CAD build for the part. Positions are in the model's coordinates, mm. A direction names the side the tool comes from. Give positions to 0.01 mm unless a question says otherwise; leave off trailing zeros. Loops run counter-clockwise (first coordinate to the right, second up) from the corner with the lowest first, then second, coordinate; pieces in that order, holes last.
Autodesk Inventor part; units mm, degrees
ref_plane "YZ Plane" through (0, 0, 0) normal (1, 0, 0) x (0, 1, 0)
ref_plane "XZ Plane" through (0, 0, 0) normal (0, 1, 0) x (-1, 0, 0)
ref_plane "XY Plane" through (0, 0, 0) normal (0, 0, 1) x (1, 0, 0)
sketch "Sketch1" plane through (0, 0, 0) normal (0, 0, 1) x (1, 0, 0)
  line L0 (-30, -3.3413) -> (15, -3.3413)
  line L1 (15, -3.3413) -> (15, -8.3413)
  line L2 (15, -8.3413) -> (-30, -8.3413)
  line L3 (-30, -8.3413) -> (-30, -3.3413)
  line L4 (-30, -65) -> (-30, 65)
  line L5 (15, -7) -> (15, 7)
  line L6 (-24.8253, -20.3413) -> (25.1747, -20.3413)
  point P0 (0, 0)
  dimension "d0" = 5
  dimension "d1" = 12
extrude "Extrusion1" add sketch "Sketch1" along normal blind 40
fillet "Fillet1" radius 5 2 edges at (-30, -5.8413, 40) (15, -5.8413, 40)
sketch "Sketch2" plane through (-30, -3.3413, 0) normal (0, 1, 0) x (1, 0, 0)
  circle A0 centre (30.1747, -28.9529) radius 2.5
  point P0 (30, 0)
hole "Hole1" at (0.1747, -3.3413, 28.9529) direction (0, -1, 0) diameter 5 depth 8 tip angle 118
sketch "Sketch3" plane through (0, 0, 0) normal (0, 0, -1) x (-1, 0, 0)
  circle A0 centre (-10, -6.5) radius 1.5
  circle A1 centre (20, -6.5) radius 1.5
  point P0 (0, 0)
hole "Hole2" at (10, -6.5, 0) at (-20, -6.5, 0) direction (0, 0, 1) diameter 2.459 depth 20 tip angle 118
properties part number "Y-Umlenkrollenhalter"
1. Saw through at C-C, the plane y = -3.9. List the corners of the cut face in (x, z), and give its area (3 significant figures).
Responses:
outline: (-30, 0) - (15, 0) - (15, 35) arc R5 ccw to (10, 40) - (-25, 40) arc R5 ccw to (-30, 35) - close; hole circle Ø5 at (0.17, 28.95)
area: 1,770 mm2
2. Drop a flat-ended pin along its axis: pin 1 (2 mm diameter, centred on x = 10, y = -6.5, fed in from -Z). Give the stop position or say it passes through.
Responses:
pin 1: stops at z = 20.14
3. Saw through at A-A, the plane x = -1. List the corners of the cut face in (y, z).
Responses:
outline: (-8.34, 0) - (-3.34, 0) - (-3.34, 26.75) - (-8.34, 26.75) - close; (-8.34, 31.16) - (-3.34, 31.16) - (-3.34, 40) - (-8.34, 40) - close
4. Saw through at D-D, the plane z = 28. List the corners of the cut face in (x, y).
Responses:
outline: (-30, -8.34) - (-2.14, -8.34) - (-2.14, -3.34) - (-30, -3.34) - close; (2.49, -8.34) - (15, -8.34) - (15, -3.34) - (2.49, -3.34) - close
5. Tool access for faces 4 (the face through (1.132, -5.876, 31.262)), 5 (the face through (-18.8, -6.77, 10.14)): list every direction of +Z, -Z, +X, -X, +Y, -Y with a clear straight run to the whole face (end or side of a thin tool).
Responses:
face 4: +Y, -Y
face 5: -Z
6. Pull direction Y, two halves, no side cores. Call faces 1 (the face through (-8, -3.341, 20)), 2 (the face through (-30, -6, 17)), 3 (the face through (10.748, -7.476, 10.14)): released by +Y, released by -Y, zero draft, split by the parting line, or undercut.
Responses:
face 1: released by +Y
face 2: zero draft
face 3: undercut
7. Saw through at B-B, the plane z = 11.5. List the corners of the cut face in (x, y).
Responses:
outline: (-30, -8.34) - (15, -8.34) - (15, -3.34) - (-30, -3.34) - close; hole circle Ø2.46 at (-20, -6.5); hole circle Ø2.46 at (10, -6.5)
8. Probe line 1 along Y through (x, z) = (10, 10); line 2 along X through (y, z) = (-6.5, 11.25); line 3 along X through (y, z) = (-3.9, 28.5). List the from-to ranges inside material, lowest first.
Responses:
line 1: y = -8.34 to -7.73, -5.27 to -3.34
line 2: x = -30 to -21.23, -18.77 to 8.77, 11.23 to 15
line 3: x = -30 to -2.28, 2.63 to 15
